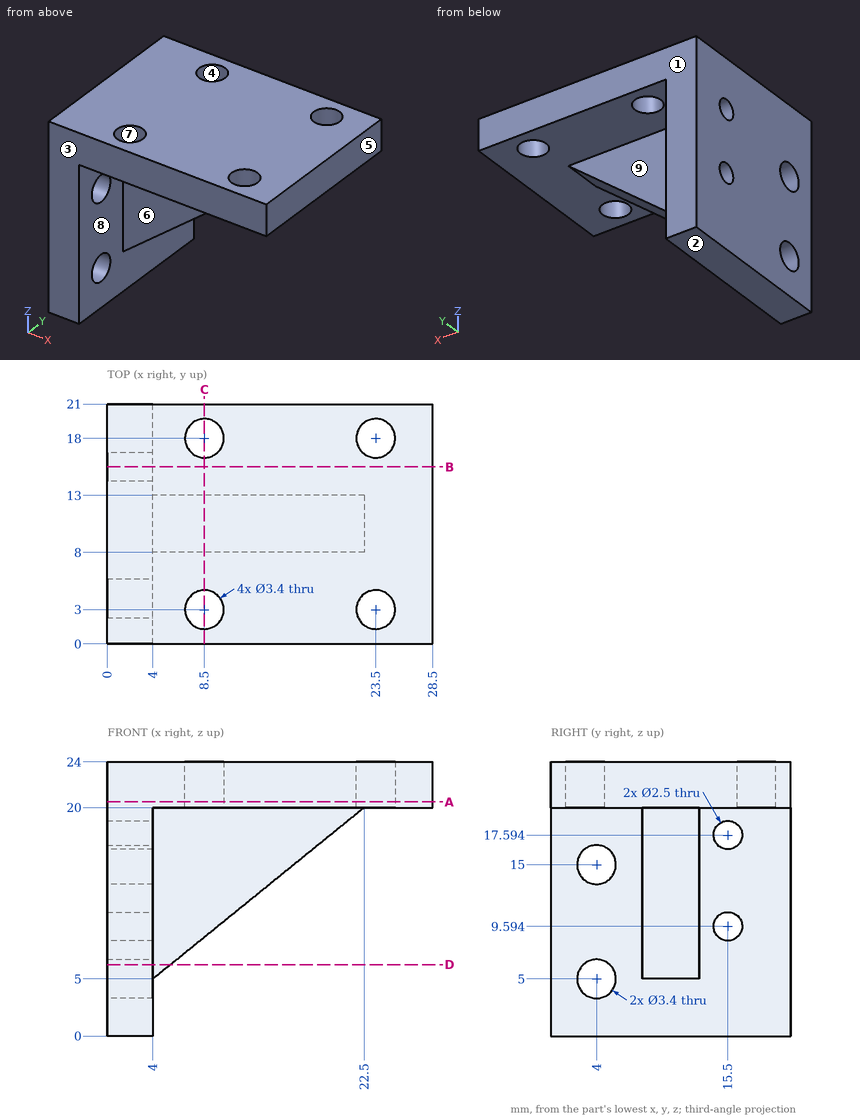
Check sheet for the drawn part. Datum: minimum x, y, z corner. Units: mm. A direction names the side the tool comes from. Coordinates: 2 decimals unless noted, no trailing zeros. Loops run counter-clockwise (first coordinate to the right, second up) from the corner with the lowest first, then second, coordinate; pieces in that order, holes last. Notation, with made-up numbers: (-32, 8) -> (19, 8) arc R28 cw to (19, 40) -> close; hole circle Ø9 at (58.25, 53). An arc over 180 degrees is marked (long way). Answer in a Markdown table with one row per item.
1) Section check A-A (z = 20.5). Record the cut outline in (x, y).
The answers:
| item | result |
|---|---|
| outline | (0, 0) -> (28.5, 0) -> (28.5, 21) -> (0, 21) -> close; hole circle Ø3.4 at (8.5, 3); hole circle Ø3.4 at (8.5, 18); hole circle Ø3.4 at (23.5, 3); hole circle Ø3.4 at (23.5, 18) |
2) Section check B-B (y = 15.5). Record the cut outline in (x, z), and give its area (3 significant figures).
The answers:
| item | result |
|---|---|
| outline | (0, 0) -> (4, 0) -> (4, 8.34) -> (0, 8.34) -> close; (0, 10.84) -> (4, 10.84) -> (4, 16.34) -> (0, 16.34) -> close; (0, 18.84) -> (4, 18.84) -> (4, 20) -> (28.5, 20) -> (28.5, 24) -> (0, 24) -> close |
| area | 174 mm2 |
3) Section check D-D (z = 6.25). Record the cut outline in (x, y), and give its area (3 significant figures).
The answers:
| item | result |
|---|---|
| outline | (0, 0) -> (4, 0) -> (4, 2.85) -> (0, 2.85) -> close; (0, 5.15) -> (4, 5.15) -> (4, 8) -> (5.54, 8) -> (5.54, 13) -> (4, 13) -> (4, 21) -> (0, 21) -> close |
| area | 82.5 mm2 |
4) Depth check by flat-ended pin: P1, Ø7.5, axis at x = 16.5, z = 11, coming from the +Y side; P2, Ø7.5, axis at x = 10, z = 15.5, coming from the -Y side; P3, Ø4.5, axis at x = 8.5, y = 18, coming from the -Z side. Enter the tip coordinate at first touch or a pass-through.
The answers:
| item | result |
|---|---|
| P1 | stops at y = 13 |
| P2 | stops at y = 8 |
| P3 | stops at z = 20 |
5) Section check C-C (x = 8.5). Record the cut outline in (y, z).
The answers:
| item | result |
|---|---|
| outline | (0, 20) -> (1.3, 20) -> (1.3, 24) -> (0, 24) -> close; (4.7, 20) -> (8, 20) -> (8, 8.65) -> (13, 8.65) -> (13, 20) -> (16.3, 20) -> (16.3, 24) -> (4.7, 24) -> close; (19.7, 20) -> (21, 20) -> (21, 24) -> (19.7, 24) -> close |
6) Access from +Z, -Z, +X, -X, +Y, -Y to the whole of each face (thin tool, end or side, straight path). Record for the marked faces 5, 6, 7, 8 and 9.
The answers:
| item | result |
|---|---|
| face 5 | +Z, -Z, +X, +Y, -Y |
| face 6 | -Z, +X, -Y |
| face 7 | +Z, -Z |
| face 8 | -Z, +X |
| face 9 | -Z, +X, +Y |
7) Draft check along Y on the marked faces 1, 2, 3 and 4. Enter one of: released by +Y, released by -Y, zero draft, split by the parting line, or undercut.
The answers:
| item | result |
|---|---|
| face 1 | released by +Y |
| face 2 | zero draft |
| face 3 | released by -Y |
| face 4 | undercut |
8) Scan lines: line 1 along Y through (x, z) = (23.5, 21.85); line 2 along Y through (x, z) = (2.1, 5); line 3 along Z through (x, y) = (5, 17.5). Record each from-to range of solid material in increasing order. Write a range as from..to.
The answers:
| item | result |
|---|---|
| line 1 | y = 0..1.3, 4.7..16.3, 19.7..21 |
| line 2 | y = 0..2.3, 5.7..21 |
| line 3 | z = 20..24 |
